```python
from build123d import *

# Parameters (mm, degrees)
F1_DEPTH = 2
F2_DEPTH = 10
F3_DEPTH = 17
F6_COUNT = 4


with BuildPart() as f1:
    # F0 (on Top) → F1 (new body)
    with BuildSketch(Plane.XY):
        with BuildLine():
            Line((0, 28.2842712475), (0, 0))
            Line((0, 0), (7, 0))
            Line((7, 0), (7, 28.2842712475))
            ThreePointArc((7, 28.2842712475), (3.5, 27.0269119346), (0, 28.2842712475))
        make_face()
    extrude(amount=F1_DEPTH)

    # F0 (on Top) → F2 (join)
    with BuildSketch(Plane.XY):
        with BuildLine():
            ThreePointArc((9, 32.5269119346), (1.1547921201, 37.5018491201), (0, 28.2842712475))
            Line((0, 28.2842712475), (0, 30.5904202615))
            ThreePointArc((0, 30.5904202615), (2.5, 36.3998952808), (7.5, 32.5269119346))
            ThreePointArc((7.5, 32.5269119346), (7.3729833462, 31.5269119346), (7, 30.5904202615))
            Line((7, 30.5904202615), (7, 28.2842712475))
            ThreePointArc((7, 28.2842712475), (8.4749371855, 30.1817040547), (9, 32.5269119346))
        make_face()
        with BuildLine():
            Line((0, 30.5904202615), (0, 28.2842712475))
            ThreePointArc((0, 28.2842712475), (3.5, 27.0269119346), (7, 28.2842712475))
            Line((7, 28.2842712475), (7, 30.5904202615))
            ThreePointArc((7, 30.5904202615), (3.5, 28.5269119346), (0, 30.5904202615))
        make_face()
    extrude(amount=F2_DEPTH)

    # F0 (on Top) → F3 (join)
    with BuildSketch(Plane.XY):
        with BuildLine():
            ThreePointArc((7.5, 32.5269119346), (2.5, 36.3998952808), (0, 30.5904202615))
            Line((0, 30.5904202615), (0, 32.5269119346))
            Line((0, 32.5269119346), (7, 32.5269119346))
            Line((7, 32.5269119346), (7, 30.5904202615))
            ThreePointArc((7, 30.5904202615), (7.3729833462, 31.5269119346), (7.5, 32.5269119346))
        make_face()
        with BuildLine():
            Line((0, 32.5269119346), (0, 30.5904202615))
            ThreePointArc((0, 30.5904202615), (3.5, 28.5269119346), (7, 30.5904202615))
            Line((7, 30.5904202615), (7, 32.5269119346))
            Line((7, 32.5269119346), (0, 32.5269119346))
        make_face()
    extrude(amount=F3_DEPTH)

    # F6: F1 ×4 about axis
    f6_axis = Axis((3.5, 0, 21.1911313236), (0, 0, 1))


with BuildPart() as f1_1:
    add(f1.part)
    for i in range(1, F6_COUNT):
        add(f1.part.rotate(f6_axis, i * 360 / F6_COUNT))


solid = f1_1.part
```
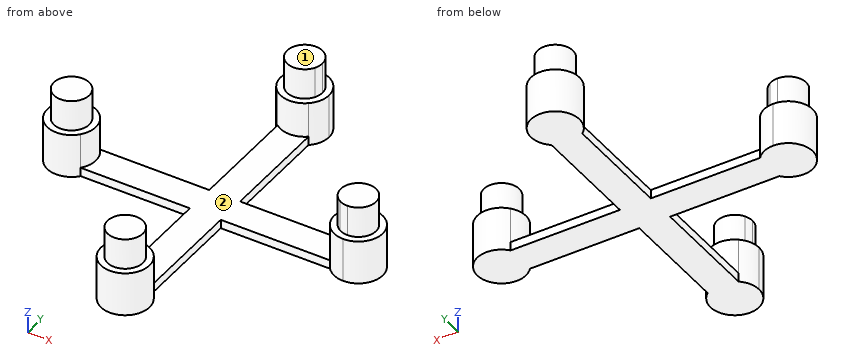
CAD build for the part. Positions are in the model's coordinates, mm. Face numbers are marked on the shaded views. Give positions to 0.01 mm unless a question says otherwise; leave off trailing zeros. Order: outer loops, then holes, each group sorted by start corner. A loop starts at its lowest first (then second) coordinate and runs counter-clockwise, first axis right, second up. Notation, with made-up numbers: M 44,-33 L 83,-33 A23 ccw 83,-9 Z; hole C 1.5,65 d2. An arc over 180 degrees is marked long. Put each result on its own line as item: value. Start each with the question number.
(1) Mould opens along Y. For the marked faces 1 and 2 say: +Y half, -Y half, draft (parallel to the pull), parting line (faces both ways), or undercut.
(2) Saw through at B-B, the plane x = 3.5. Write the cut outline in (y, z), then the cut area to 3 significant figures.
(3) Saw through at D-D, the plane z = 5.5. Write the cut outline in (x, y).
(4) Saw through at A-A, the plane z = 13.5. Write the cut outline in (x, y), then the cut area to 3 significant figures.
(5) Flat gauge pins, fed straight in: pin 1 Ø4 at (x, z) = (-23, 6.5) entering from -Y; pin 2 Ø0.6 at (x, z) = (15.5, 1.5) entering from -Y; pin 3 Ø2 at (x, z) = (-15, 1) entering from +Y. Where does each tip first touch, or does it go through?
(6) Saw through at C-C, the plane y = 0. Write the cut outline in (x, z), then the cut area to 3 significant figures.
(7) Drill centre lines: line 1 along Y through (x, z) = (15, 1.5); line 2 along Z through (x, y) = (6.5, -25); line 3 along Y through (x, z) = (-29, 13.5). Where is each one in solid material? Low to high.
Check result:
1. face 1: draft
1. face 2: undercut
2. outline: M -38.03,0 L 38.03,0 L 38.03,10 L 36.53,10 L 36.53,17 L 28.53,17 L 28.53,10 L 27.03,10 L 27.03,2 L -27.03,2 L -27.03,10 L -28.53,10 L -28.53,17 L -36.53,17 L -36.53,10 L -38.03,10 Z
2. area: 440 mm2
3. outline: C -29.03,0 d11; C 3.5,-32.53 d11; C 3.5,32.53 d11; C 36.03,0 d11
4. outline: C -29.03,0 d8; C 3.5,-32.53 d8; C 3.5,32.53 d8; C 36.03,0 d8
4. area: 201 mm2
5. pin 1: stops at y = -3.75
5. pin 2: stops at y = -3.5
5. pin 3: stops at y = 3.5
6. outline: M -34.53,0 L 41.53,0 L 41.53,10 L 40.03,10 L 40.03,17 L 32.03,17 L 32.03,10 L 30.53,10 L 30.53,2 L -23.53,2 L -23.53,10 L -25.03,10 L -25.03,17 L -33.03,17 L -33.03,10 L -34.53,10 Z
6. area: 440 mm2
7. line 1: y = -3.5 to 3.5
7. line 2: z = 0 to 2
7. line 3: y = -4 to 4
